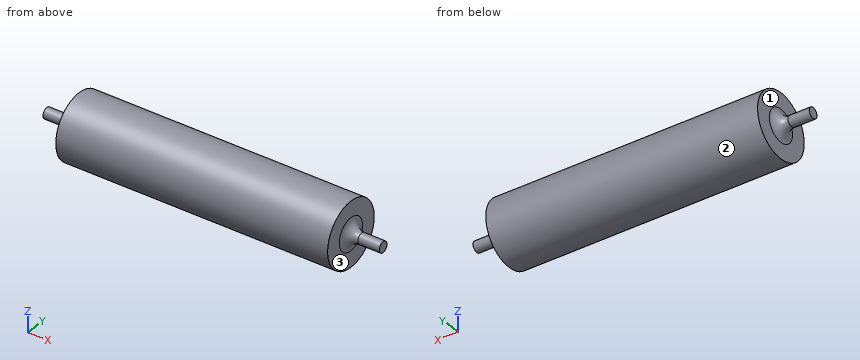
from build123d import *

# Parameters (mm, degrees)
CONG_1_R = 5


with BuildPart() as part:
    # Esquisse1 → Révolution1 (revolve)
    with BuildSketch(Plane.XY, mode=Mode.PRIVATE) as r_volution1_sk:
        Polygon((-78.3, 0), (-78.3, 2.5), (-63.3, 2.5), (-63.3, 15), (63.3, 15), (63.3, 2.5), (78.3, 2.5), (78.3, 0), align=None)
    revolve(r_volution1_sk.sketch.rotate(Axis((-78.3, 0, 0), (1, 0, 0)), 180), axis=Axis((-78.3, 0, 0), (1, 0, 0)))

    # Congé1
    cong_1_edges = [part.edges().sort_by_distance(p)[0] for p in [
        (-63.3, 2.5, 0),
        (63.3, 2.5, 0),
    ]]
    fillet(cong_1_edges, radius=CONG_1_R)


solid = part.part
The listing builds one solid part. Answer for the finished solid, in the listing's coordinates (mm). Face numbers are marked on the shaded views. A direction names the side the tool comes from. Round coordinates to 2 decimals unless told otherwise and drop trailing zeros. Order: outer loops, then holes, each group sorted by start corner. A loop starts at its lowest first (then second) coordinate and runs counter-clockwise, first axis right, second up. Notation, with made-up numbers: M 36,-2.5 L 50,-2.5 A8 ccw 50,6.5 Z; hole C 80.5,69 d10. An arc over 180 degrees is marked long. Answer in a Markdown table with one row per item. Add a question column.
1) The part is cut by section B-B on x = 26.5. Determine the outline of the cut face in (y, z).
2) The part is cut by section C-C on y = -10.75. Determine the outline of the cut face in (x, z), plus the area to 3 significant figures.
3) The part is cut by section A-A on y = 0. Determine the outline of the cut face in (x, z).
4) Flat-ended cylindrical pins translate along their axes: pin 1 Ø2 at (y, z) = (-9.5, 10) entering from -X; pin 2 Ø2 at (x, y) = (40, -7.5) entering from +Z; pin 3 Ø8 at (y, z) = (-2.5, -6.5) entering from +X. Find the tip coordinate at first contact, or state that the pin passes through.
5) Which of the six approach directions +Z, -Z, +X, -X, +Y, -Y give full straight-line access (tool end or side, diameter ignored) to the marked faces 1, 2 and 3?
6) Consider line 1 along X through (y, z) = (1.25, -8.5); line 2 along Z through (x, y) = (59, 8.75); line 3 along Y through (x, z) = (-54.5, -4.25). Determine where each line is inside the solid, lowest interval first. Write a range as from..to.
Findings below:
| question | item | result |
|---|---|---|
| 1 | outline | C 0,0 d30 |
| 2 | outline | M -63.3,-10.46 L 63.3,-10.46 L 63.3,10.46 L -63.3,10.46 Z |
| 2 | area | 2,650 mm² |
| 3 | outline | M -78.3,-2.5 L -68.3,-2.5 A5 cw -63.3,-7.5 L -63.3,-15 L 63.3,-15 L 63.3,-7.5 A5 cw 68.3,-2.5 L 78.3,-2.5 L 78.3,2.5 L 68.3,2.5 A5 cw 63.3,7.5 L 63.3,15 L -63.3,15 L -63.3,7.5 A5 cw -68.3,2.5 L -78.3,2.5 Z |
| 4 | pin 1 | stops at x = -63.3 |
| 4 | pin 2 | stops at z = 13.52 |
| 4 | pin 3 | stops at x = 66.2 |
| 5 | face 1 | -X |
| 5 | face 2 | +X, -X |
| 5 | face 3 | +X |
| 6 | line 1 | x = -63.3..63.3 |
| 6 | line 2 | z = -12.18..12.18 |
| 6 | line 3 | y = -14.39..14.39 |
